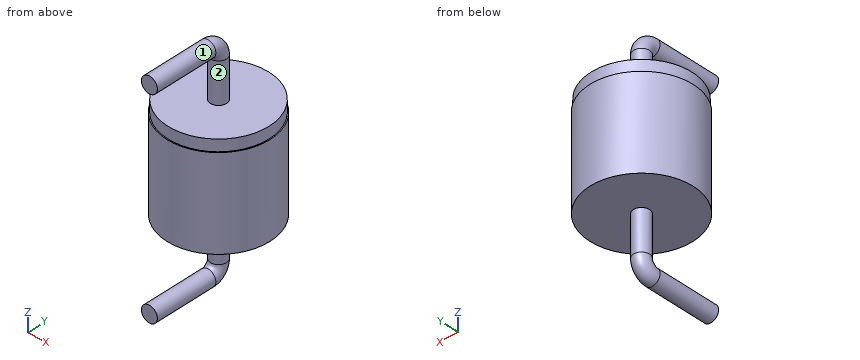
from build123d import *

# Parameters (mm, degrees)
SKETCH_1_R          = 4.5
EXTRUDE_1_DEPTH     = 4.5
SKETCH_2_R          = 5.333427414
SKETCH_2_R_2        = 4.410947686
CUT_EXTRUDE_1_DEPTH = 1
SKETCH_4_R          = 0.7


with BuildPart() as part:
    # Эскиз1 → Бобышка-Вытянуть1 (new, symmetric)
    with BuildSketch(Plane.XY):
        Circle(SKETCH_1_R)
    extrude(amount=EXTRUDE_1_DEPTH, both=True)

    # Эскиз2 → Вырез-Вытянуть1 (cut)
    with BuildSketch(Plane.XY.offset(4.5)):
        Circle(SKETCH_2_R)
        Circle(SKETCH_2_R_2, mode=Mode.SUBTRACT)
    extrude(amount=-CUT_EXTRUDE_1_DEPTH, mode=Mode.SUBTRACT)

    # По траектории1: sweep along a path in Эскиз3
    with BuildLine(Plane(origin=(0, 0, 0), x_dir=(0, 0, -1), z_dir=(1, 0, 0))) as sweep_1_path:
        Line((9, -6.5), (9, -1))
        ThreePointArc((9, -1), (8.707106781, -0.292893219), (8, 0))
        Line((8, 0), (-8, 0))
        ThreePointArc((-8, 0), (-8.707106781, -0.292893219), (-9, -1))
        Line((-9, -1), (-9, -6.5))
    # Эскиз4 → По траектории1 (sweep)
    with BuildSketch(Plane.XY):
        Circle(SKETCH_4_R)
    sweep(path=sweep_1_path.line)


solid = part.part
CAD build for the part. Positions are in the model's coordinates, mm. Face numbers are marked on the shaded views. A direction names the side the tool comes from. Round coordinates to 2 decimals unless told otherwise and drop trailing zeros. Loops run counter-clockwise (first coordinate to the right, second up) from the corner with the lowest first, then second, coordinate; pieces in that order, holes last. Notation, with made-up numbers: (68, 4) - (121, 4) arc R24 ccw to (121, 17) - close; hole circle Ø7 at (69, 2.25). An arc over 180 degrees is marked (long way). Put each result on its own line as item: value.
1. Slice it at B-B on y = -6. List the corners of the cut face in (x, z).
Geometry check:
outline: circle Ø1.4 at (0, -9); circle Ø1.4 at (0, 9)
2. Slice it at A-A on x = 0. List the corners of the cut face in (y, z).
Geometry check:
outline: (-6.5, -9.7) - (-1, -9.7) arc R1.7 ccw to (0.7, -8) - (0.7, -4.5) - (4.5, -4.5) - (4.5, 3.5) - (4.41, 3.5) - (4.41, 4.5) - (0.7, 4.5) - (0.7, 8) arc R1.7 ccw to (-1, 9.7) - (-6.5, 9.7) - (-6.5, 8.3) - (-1, 8.3) arc R0.3 cw to (-0.7, 8) - (-0.7, 4.5) - (-4.41, 4.5) - (-4.41, 3.5) - (-4.5, 3.5) - (-4.5, -4.5) - (-0.7, -4.5) - (-0.7, -8) arc R0.3 cw to (-1, -8.3) - (-6.5, -8.3) - close
3. Wall check: line 1 (Z direction, x = 3.5, y = -1.25); line 2 (X direction, y = -1.25, z = 1); line 3 (Y direction, x = 0.25, z = -7.25). Give the ranges that are in metal, low to high.
Geometry check:
line 1: -4.5 to 4.5
line 2: -4.32 to 4.32
line 3: -0.65 to 0.65
4. Slice it at C-C on y = -2.5. List the corners of the cut face in (x, z).
Geometry check:
outline: (-3.74, -4.5) - (3.74, -4.5) - (3.74, 3.5) - (3.63, 3.5) - (3.63, 4.5) - (-3.63, 4.5) - (-3.63, 3.5) - (-3.74, 3.5) - close; circle Ø1.4 at (0, -9); circle Ø1.4 at (0, 9)
5. Slice it at D-D on y = 2. List the corners of the cut face in (x, z).
Geometry check:
outline: (-4.03, -4.5) - (4.03, -4.5) - (4.03, 3.5) - (3.93, 3.5) - (3.93, 4.5) - (-3.93, 4.5) - (-3.93, 3.5) - (-4.03, 3.5) - close
6. 3-axis set-ups, long thin cutter, end or side, ignore diameter. For the marked faces 1 and 2: which of +Z, -Z, +X, -X, +Y, -Y reach the whole face in a straight line?
Geometry check:
face 1: -Y
face 2: none
7. Pin check, flat tips, straight feed: P1, Ø3, axis at y = -5, z = 6, coming from the +X side; P2, Ø1.5, axis at y = -1, z = 4, coming from the -X side; P3, Ø3, axis at x = -1, z = 7.5, coming from the +Y side. Stop position of each tip, or through.
Geometry check:
P1: through
P2: x = -4.48
P3: y = 0.7
